from build123d import *

# Parameters (mm, degrees)
F0_W     = 40
F0_H     = 40
F0_W_2   = 32.8
F0_H_2   = 32.8
F1_DEPTH = 25
F2_W     = 11.8
F2_H     = 16.8
F2_W_2   = 3.8
F2_H_2   = 8.8
F3_DEPTH = 25
F4_W     = 40
F4_H     = 40
F4_W_2   = 3.8
F4_H_2   = 8.8
F5_DEPTH = 0.9


with BuildPart() as f1:
    # F0 (on Top) → F1 (new body)
    with BuildSketch(Plane.XY):
        Rectangle(F0_W, F0_H)
        Rectangle(F0_W_2, F0_H_2, mode=Mode.SUBTRACT)
    extrude(amount=F1_DEPTH)



with BuildPart() as f3:
    # F2 (on Top) → F3 (new body)
    with BuildSketch(Plane.XY):
        Rectangle(F2_W, F2_H)
        Rectangle(F2_W_2, F2_H_2, mode=Mode.SUBTRACT)
    extrude(amount=F3_DEPTH)


with BuildPart() as f1_1:
    add(f1.part)

    add(f3.part)  # F5 merges F3
    # F4 (on face) → F5 (join)
    with BuildSketch(Plane(origin=(0, 0, 0), x_dir=(1, 0, 0), z_dir=(0, 0, -1))):
        Rectangle(F4_W, F4_H)
        Rectangle(F4_W_2, F4_H_2, mode=Mode.SUBTRACT)
    extrude(amount=F5_DEPTH)


solid = f1_1.part
Input: part model. Units: mm. Frame: model coordinates. A direction names the side the tool comes from. Give positions to 0.01 mm unless a question says otherwise; leave off trailing zeros. Write each loop counter-clockwise with the first axis right and the second up, starting at its lowest first coordinate (ties: lowest second). Pieces come first, ordered by that corner, then holes. Notation, with made-up numbers: M -33.75,22 L 9.25,22 A30 cw 9.25,56 Z; hole C 22,-29.75 d8. An arc over 180 degrees is marked long. Write item = value, one per line. Start each with the question number.
1) Reachability of faces 1 (the flat face through (-1.9, 0, 12)), 2 (the flat face through (0, -8.4, 12)), 3 (the flat face through (0, 20, 12)) from +Z, -Z, +X, -X, +Y, -Y: full face, straight path, thin tool, end or side. Return the list, or none.
2) Cut plane C-C on x = 0.5. Return the cut outline in (y, z).
3) Material intervals for line 1 along X through (y, z) = (-5, 8); line 2 along X through (y, z) = (-2, 2); line 3 along Y through (x, z) = (-2, 15.5), sorted ascending. Write a range as [from, to].
4) Draft query along Y for faces 4 (the flat face through (-18, 0, 25)), 5 (the flat face through (1.9, 0, 12)), 6 (the flat face through (0, -20, 12)). Return one class per face: +Y half, -Y half, draft (parallel to the pull), parting line (faces both ways), or undercut.
5) Cut plane B-B on y = 2. Return the cut outline in (x, z), then the cut area to 3 significant figures.
6) Cut plane A-A on z = 5. Return the cut outline in (x, y).
7) Cut plane D-D on y = 12.5. Return the cut outline in (x, z).
Solved:
q1.face_1 = +Z, -Z
q1.face_2 = +Z
q1.face_3 = +Z, -Z, +X, -X, +Y
q2.outline = M -20,-0.9 L -4.4,-0.9 L -4.4,25 L -8.4,25 L -8.4,0 L -16.4,0 L -16.4,25 L -20,25 Z; M 4.4,-0.9 L 20,-0.9 L 20,25 L 16.4,25 L 16.4,0 L 8.4,0 L 8.4,25 L 4.4,25 Z
q3.line_1 = [-20, -16.4], [-5.9, 5.9], [16.4, 20]
q3.line_2 = [-20, -16.4], [-5.9, -1.9], [1.9, 5.9], [16.4, 20]
q3.line_3 = [-20, -16.4], [-8.4, 8.4], [16.4, 20]
q4.face_4 = draft
q4.face_5 = undercut
q4.face_6 = -Y half
q5.outline = M -20,-0.9 L -1.9,-0.9 L -1.9,25 L -5.9,25 L -5.9,0 L -16.4,0 L -16.4,25 L -20,25 Z; M 1.9,-0.9 L 20,-0.9 L 20,25 L 16.4,25 L 16.4,0 L 5.9,0 L 5.9,25 L 1.9,25 Z
q5.area = 413 mm2
q6.outline = M -20,-20 L 20,-20 L 20,20 L -20,20 Z; M -5.9,-8.4 L 5.9,-8.4 L 5.9,8.4 L -5.9,8.4 Z; hole M -16.4,-16.4 L 16.4,-16.4 L 16.4,16.4 L -16.4,16.4 Z; hole M -1.9,-4.4 L 1.9,-4.4 L 1.9,4.4 L -1.9,4.4 Z
q7.outline = M -20,-0.9 L 20,-0.9 L 20,25 L 16.4,25 L 16.4,0 L -16.4,0 L -16.4,25 L -20,25 Z
